Read the model definition and answer for the solid it produces. Units are mm, in the model's axes. Round coordinates to 2 decimals unless told otherwise and drop trailing zeros. Loops run counter-clockwise (first coordinate to the right, second up) from the corner with the lowest first, then second, coordinate; pieces in that order, holes last. Notation, with made-up numbers: (2.5, 85) - (34.5, 85) arc R22 cw to (34.5, 124) - close; hole circle Ø7 at (43, -5.5). An arc over 180 degrees is marked (long way). Use one line per item in the form item = value. Start each with the question number.
Autodesk Inventor part; units mm, degrees
ref_plane "YZ Plane" through (0, 0, 0) normal (1, 0, 0) x (0, 1, 0)
ref_plane "XZ Plane" through (0, 0, 0) normal (0, 1, 0) x (-1, 0, 0)
ref_plane "XY Plane" through (0, 0, 0) normal (0, 0, 1) x (1, 0, 0)
sketch "Sketch7" plane through (0, 0, 0) normal (0, 1, 0) x (-1, 0, 0)
  line L0 (5, 0) -> (25, 0)
  line L1 (30, 5) -> (30, 150)
  line L2 (25, 150) -> (5, 150)
  line L3 (0, 145) -> (0, 5)
  line L4 (30, 145) -> (30, 145)
  line L5 (30, 145) -> (22.5, 145)
  circle A0 centre (22.5, 145) radius 2.75
  circle A1 centre (22.5, 130) radius 2.75
  circle A2 centre (7.5, 145) radius 2.75
  circle A3 centre (7.5, 130) radius 2.75
  line L6 (22.5, 130) -> (30, 130)
  line L7 (30, 130) -> (30, 125)
  circle A4 centre (22.5, 35) radius 2.75
  circle A5 centre (22.5, 5) radius 2.75
  circle A6 centre (7.5, 35) radius 2.75
  circle A7 centre (7.5, 5) radius 2.75
  circle A8 centre (22.5, 115) radius 2.75
  circle A9 centre (7.5, 115) radius 2.75
  circle A10 centre (22.5, 100) radius 2.75
  circle A11 centre (7.5, 100) radius 2.75
  arc A12 (30, 145) -> (25, 150) centre (25, 145) ccw
  arc A13 (5, 150) -> (0, 145) centre (5, 145) ccw
  arc A14 (25, 0) -> (30, 5) centre (25, 5) ccw
  arc A15 (0, 5) -> (5, 0) centre (5, 5) ccw
  point P0 (0, 0)
  point P1 (30, 0)
  point P2 (0, 150)
  dimension "d141" = 30
  dimension "d142" = 150
  dimension "d143" = 5
  dimension "d144" = 7.5
  dimension "d145" = 5.5
  dimension "d148" = 15
  dimension "d151" = 15
  dimension "d154" = 5
  dimension "d159" = 5.5
  dimension "d160" = 30
  dimension "d161" = 15
  dimension "d162" = 5
extrude "Extrusion5" add sketch "Sketch7" along normal blind 6
properties part number "GARFO" material "Aluminium AW-7020"
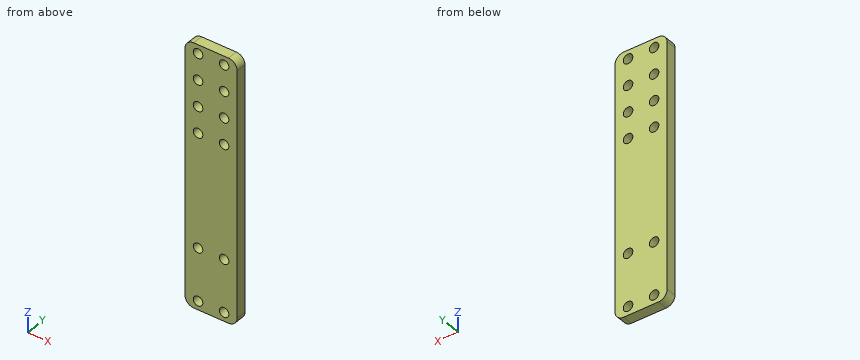
1) Straight lines are drawn through the part: line 1 (X direction, y = 4.7, z = 130); line 2 (Z direction, x = -2, y = 4.9); line 3 (Z direction, x = -1.25, y = 1.75). For each, find the intervals that lie inside material, in ascending order. Write a range as from..to.
2) A cutting plane is placed at C-C on y = 4.1. Count the separate pieces of the cut face and the enclosed holes in it, plus the area to 3 significant figures.
3) A cutting plane is placed at B-B on z = 100. Write down the section's boundary in (x, y).
4) A cutting plane is placed at D-D on x = -23.5. Write down the section's boundary in (y, z).
5) A cutting plane is placed at A-A on x = -7.5. Write down the section's boundary in (y, z).
6) A flat-ended cylindrical pin translates along its axis: pin 1 (1 mm diameter, centred on x = -3.5, y = 4, fed in from +Z). Find the tip coordinate at first contact, or state that the pin passes through.
Checks:
q1.line_1 = -30..-25.25, -19.75..-10.25, -4.75..0
q1.line_2 = 1..149
q1.line_3 = 1.69..148.31
q2.separate_pieces = 1
q2.enclosed_holes = 12
q2.area = 4,190 mm²
q3.outline = (-30, 0) - (-25.25, 0) - (-25.25, 6) - (-30, 6) - close; (-19.75, 0) - (-10.25, 0) - (-10.25, 6) - (-19.75, 6) - close; (-4.75, 0) - (0, 0) - (0, 6) - (-4.75, 6) - close
q4.outline = (0, 0) - (6, 0) - (6, 2.44) - (0, 2.44) - close; (0, 7.56) - (6, 7.56) - (6, 32.44) - (0, 32.44) - close; (0, 37.56) - (6, 37.56) - (6, 97.44) - (0, 97.44) - close; (0, 102.56) - (6, 102.56) - (6, 112.44) - (0, 112.44) - close; (0, 117.56) - (6, 117.56) - (6, 127.44) - (0, 127.44) - close; (0, 132.56) - (6, 132.56) - (6, 142.44) - (0, 142.44) - close; (0, 147.56) - (6, 147.56) - (6, 150) - (0, 150) - close
q5.outline = (0, 0) - (6, 0) - (6, 2.25) - (0, 2.25) - close; (0, 7.75) - (6, 7.75) - (6, 32.25) - (0, 32.25) - close; (0, 37.75) - (6, 37.75) - (6, 97.25) - (0, 97.25) - close; (0, 102.75) - (6, 102.75) - (6, 112.25) - (0, 112.25) - close; (0, 117.75) - (6, 117.75) - (6, 127.25) - (0, 127.25) - close; (0, 132.75) - (6, 132.75) - (6, 142.25) - (0, 142.25) - close; (0, 147.75) - (6, 147.75) - (6, 150) - (0, 150) - close
q6.pin_1 = 149.9
